from build123d import *

# Parameters (mm, degrees)
SKETCH_2_R          = 2.55
EXTRUDE_1_DEPTH     = 205
SKETCH_3_R          = 3
CUT_EXTRUDE_1_DEPTH = 207.215906273


with BuildPart() as part:
    # 草图2 → 凸台-拉伸1 (new body)
    with BuildSketch(Plane.XY):
        with BuildLine():
            Line((-3.9, 2.839339828), (-6.560660172, 5.5))
            Line((-6.560660172, 5.5), (-8.2, 5.5))
            Line((-8.2, 5.5), (-8.2, 3.1))
            Line((-8.2, 3.1), (-9.45, 3.1))
            Line((-9.45, 3.1), (-9.45, 3.65))
            Line((-9.45, 3.65), (-10, 3.65))
            Line((-10, 3.65), (-10, 8.5))
            ThreePointArc((-10, 8.5), (-9.560660172, 9.560660172), (-8.5, 10))
            Line((-8.5, 10), (-3.65, 10))
            Line((-3.65, 10), (-3.65, 9.45))
            Line((-3.65, 9.45), (-3.1, 9.45))
            Line((-3.1, 9.45), (-3.1, 8.2))
            Line((-3.1, 8.2), (-5.5, 8.2))
            Line((-5.5, 8.2), (-5.5, 6.560660172))
            Line((-5.5, 6.560660172), (-2.839339828, 3.9))
            Line((-2.839339828, 3.9), (2.839339828, 3.9))
            Line((2.839339828, 3.9), (5.5, 6.560660172))
            Line((5.5, 6.560660172), (5.5, 8.2))
            Line((5.5, 8.2), (3.1, 8.2))
            Line((3.1, 8.2), (3.1, 9.45))
            Line((3.1, 9.45), (3.65, 9.45))
            Line((3.65, 9.45), (3.65, 10))
            Line((3.65, 10), (8.5, 10))
            ThreePointArc((8.5, 10), (9.560660172, 9.560660172), (10, 8.5))
            Line((10, 8.5), (10, 3.65))
            Line((10, 3.65), (9.45, 3.65))
            Line((9.45, 3.65), (9.45, 3.1))
            Line((9.45, 3.1), (8.2, 3.1))
            Line((8.2, 3.1), (8.2, 5.5))
            Line((8.2, 5.5), (6.560660172, 5.5))
            Line((6.560660172, 5.5), (3.9, 2.839339828))
            Line((3.9, 2.839339828), (3.9, -2.839339828))
            Line((3.9, -2.839339828), (6.560660172, -5.5))
            Line((6.560660172, -5.5), (8.2, -5.5))
            Line((8.2, -5.5), (8.2, -3.1))
            Line((8.2, -3.1), (9.45, -3.1))
            Line((9.45, -3.1), (9.45, -3.65))
            Line((9.45, -3.65), (10, -3.65))
            Line((10, -3.65), (10, -8.5))
            ThreePointArc((10, -8.5), (9.560660172, -9.560660172), (8.5, -10))
            Line((8.5, -10), (3.65, -10))
            Line((3.65, -10), (3.65, -9.45))
            Line((3.65, -9.45), (3.1, -9.45))
            Line((3.1, -9.45), (3.1, -8.2))
            Line((3.1, -8.2), (5.5, -8.2))
            Line((5.5, -8.2), (5.5, -6.560660172))
            Line((5.5, -6.560660172), (2.839339828, -3.9))
            Line((2.839339828, -3.9), (-2.839339828, -3.9))
            Line((-2.839339828, -3.9), (-5.5, -6.560660172))
            Line((-5.5, -6.560660172), (-5.5, -8.2))
            Line((-5.5, -8.2), (-3.1, -8.2))
            Line((-3.1, -8.2), (-3.1, -9.45))
            Line((-3.1, -9.45), (-3.65, -9.45))
            Line((-3.65, -9.45), (-3.65, -10))
            Line((-3.65, -10), (-8.5, -10))
            ThreePointArc((-8.5, -10), (-9.560660172, -9.560660172), (-10, -8.5))
            Line((-10, -8.5), (-10, -3.65))
            Line((-10, -3.65), (-9.45, -3.65))
            Line((-9.45, -3.65), (-9.45, -3.1))
            Line((-9.45, -3.1), (-8.2, -3.1))
            Line((-8.2, -3.1), (-8.2, -5.5))
            Line((-8.2, -5.5), (-6.560660172, -5.5))
            Line((-6.560660172, -5.5), (-3.9, -2.839339828))
            Line((-3.9, -2.839339828), (-3.9, 2.839339828))
        make_face()
        with Locations(Location((0, 0, 0), (0, 0, 180))):
            Circle(SKETCH_2_R, mode=Mode.SUBTRACT)
    extrude(amount=EXTRUDE_1_DEPTH)

    # 草图3 → 切除-拉伸1 (cut, through all)
    with BuildSketch(Plane.XZ.offset(10)):
        with Locations(Location((0, 167.5, 0), (0, 0, 198.835996158))):
            Circle(SKETCH_3_R)
        with Locations(Location((0, 37.5, 0), (0, 0, 198.835996158))):
            Circle(SKETCH_3_R)
    extrude(amount=-CUT_EXTRUDE_1_DEPTH, mode=Mode.SUBTRACT)


solid = part.part
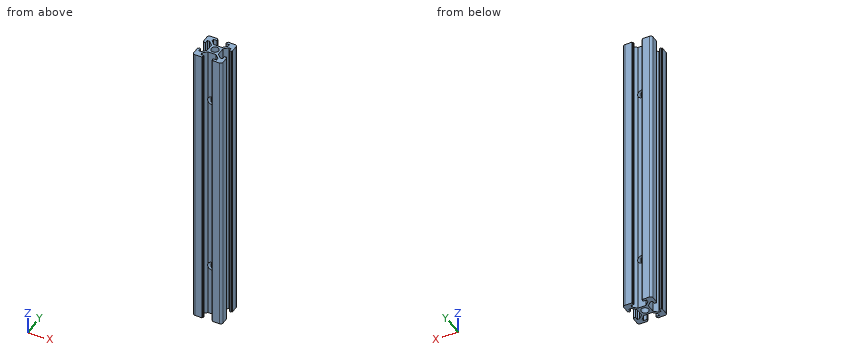
Work out the finished part from the listing and answer in its coordinate system (mm). Coordinates: 2 decimals unless noted, no trailing zeros. Write each loop counter-clockwise with the first axis right and the second up, starting at its lowest first coordinate (ties: lowest second). Pieces come first, ordered by that corner, then holes.
1. Consider line 1 along Y through (x, z) = (0, 193.5); line 2 along X through (y, z) = (-4.5, 115.5); line 3 along Y through (x, z) = (-3.5, 9). Determine where each line is inside the solid, lowest interval first.
Results list:
line 1: y = -3.9 to -2.55, 2.55 to 3.9
line 2: x = -10 to -8.2, -5.56 to -3.44, 3.44 to 5.56, 8.2 to 10
line 3: y = -9.45 to -8.2, -4.56 to 4.56, 8.2 to 9.45
2. The part is cut by section A-A, the plane y = 0. Write down the section's boundary in (x, z), and give its area (3 significant figures).
Results list:
outline: (-3.9, 0) - (-2.55, 0) - (-2.55, 35.92) arc R3 cw to (-2.55, 39.08) - (-2.55, 165.92) arc R3 cw to (-2.55, 169.08) - (-2.55, 205) - (-3.9, 205) - close; (2.55, 0) - (3.9, 0) - (3.9, 205) - (2.55, 205) - (2.55, 169.08) arc R3 cw to (2.55, 165.92) - (2.55, 39.08) arc R3 cw to (2.55, 35.92) - close
area: 550 mm2
3. The part is cut by section B-B, the plane x = 0. Write down the section's boundary in (y, z).
Results list:
outline: (-3.9, 0) - (-2.55, 0) - (-2.55, 34.5) - (-3.9, 34.5) - close; (-3.9, 40.5) - (-2.55, 40.5) - (-2.55, 164.5) - (-3.9, 164.5) - close; (-3.9, 170.5) - (-2.55, 170.5) - (-2.55, 205) - (-3.9, 205) - close; (2.55, 0) - (3.9, 0) - (3.9, 34.5) - (2.55, 34.5) - close; (2.55, 40.5) - (3.9, 40.5) - (3.9, 164.5) - (2.55, 164.5) - close; (2.55, 170.5) - (3.9, 170.5) - (3.9, 205) - (2.55, 205) - close
4. Flat-ended cylindrical pins translate along their axes: pin 1 (6 mm diameter, centred on x = -0.5, z = 192.5, fed in from +Y); pin 2 (4 mm diameter, centred on x = 1, z = 158, fed in from -Y); pin 3 (0.6 mm diameter, centred on y = 9.5, z = 100.5, fed in from -X). Find the tip coordinate at first contact, or state that the pin passes through.
Results list:
pin 1: stops at y = 9.45
pin 2: stops at y = -4.06
pin 3: stops at x = -9.83
